Could you check a few things on this model? Use its own coordinates, in mm. Face numbers are marked on the shaded views. A direction names the side the tool comes from. Give positions to 0.01 mm unless a question says otherwise; leave off trailing zeros. Order: outer loops, then holes, each group sorted by start corner. A loop starts at its lowest first (then second) coordinate and runs counter-clockwise, first axis right, second up. Notation, with made-up numbers: (-1, -13.5) -> (42, -13.5) arc R28 cw to (42, 18.5) -> close; hole circle Ø4 at (-13.75, 62). An arc over 180 degrees is marked (long way). Answer as CSV lines item,"result". Start each with the question number.
(1) We'd pull the mould along X, two halves only. Please class the marked faces 1, 2 and 3: released by +X, released by -X, zero draft, split by the parting line, or undercut.
(2) On a 3-axis mill with a long thin cutter (end or side, diameter ignored), from which of +Z, -Z, +X, -X, +Y, -Y can I reach the whole of each face in a straight line? I mean the marked faces 4, 5 and 6. Say none if no direction works.
(3) Will these pins go through, and if not, where does the flat tip stop? pin 1 Ø14 at (y, z) = (-46.5, 30.5) entering from -X; pin 2 Ø1 at (x, y) = (91.5, -16.5) entering from +Z; pin 3 Ø3 at (x, z) = (57, 42) entering from +Y.
(4) I want a section at B-B (y = -7). Please give me the cut outline in (x, z).
(5) I want a section at C-C (z = 44.5). Please give me the cut outline in (x, y).
(6) I need wall thicknesses on L1, parallel to Z at x = 25.4, y = -32.75 (3 decimals); L2, parallel to Y at x = 40, z = 15.5; L3, parallel to X at y = -4, z = 17. Which ranges of each line are inside material? Lowest first, please.
(7) I want a section at D-D (x = 118). Please give me the cut outline in (y, z).
(8) I want a section at A-A (x = 18). Please give me the cut outline in (y, z).
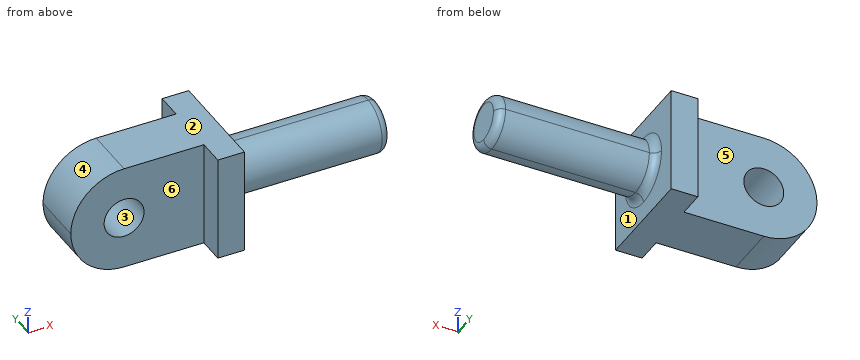
```python
from build123d import *

# Parameters (mm, degrees)
F0_W     = 76.2
F0_H     = 50.8
F1_DEPTH = 50.8
F2_W     = 63.5
F2_H     = 12.7
F3_DEPTH = 177.8
F5_DEPTH = 127
F6_R     = 25.39999
F8_DEPTH = 76.2
F9_R     = 3.81


# Not quite as in the source:
# - a fillet or chamfer is up to 0.001 mm smaller than in the source, because OpenCascade refuses the exact size


with BuildPart() as f1:
    # F0 (on Front) → F1 (new body)
    with BuildSketch(Plane.XZ):
        with Locations((38.1, 25.4)):
            Rectangle(F0_W, F0_H)
    extrude(amount=F1_DEPTH)

    # F2 (on face) → F3 (cut)
    with BuildSketch(Plane.XY.offset(50.8)):
        with Locations((31.75, -6.35)):
            Rectangle(F2_W, F2_H)
        with Locations((31.75, -44.45)):
            Rectangle(F2_W, F2_H)
    extrude(amount=-F3_DEPTH, mode=Mode.SUBTRACT)

    # F4 (on face) → F5 (cut)
    with BuildSketch(Plane.XZ.offset(38.1)):
        with BuildLine():
            ThreePointArc((15.875, 25.4), (25.4, 15.875), (34.925, 25.4))
            ThreePointArc((34.925, 25.4), (25.4, 34.925), (15.875, 25.4))
        make_face()
    extrude(amount=-F5_DEPTH, mode=Mode.SUBTRACT)

    # F6 (radius 25.4 in the source; OpenCascade refuses exactly that, so slightly less here)
    f6_edges = [f1.edges().sort_by_distance(p)[0] for p in [
        (0, -25.4, 0),
        (0, -25.4, 50.8),
    ]]
    fillet(f6_edges, radius=F6_R)

    # F7 (on face) → F8 (join)
    with BuildSketch(Plane.YZ.offset(76.2)):
        with BuildLine():
            ThreePointArc((-12.7, 25.4), (-16.4197438789, 34.3802561211), (-25.4, 38.1))
            Line((-25.4, 38.1), (-25.4, 12.7))
            ThreePointArc((-25.4, 12.7), (-16.4197438789, 16.4197438789), (-12.7, 25.4))
        make_face()
        with BuildLine():
            Line((-25.4, 12.7), (-25.4, 38.1))
            ThreePointArc((-25.4, 38.1), (-38.1, 25.4), (-25.4, 12.7))
        make_face()
    extrude(amount=F8_DEPTH)

    # F9
    f9_edges = [f1.edges().sort_by_distance(p)[0] for p in [
        (152.4, -38.1, 25.4),
        (76.2, -38.1, 25.4),
    ]]
    fillet(f9_edges, radius=F9_R)


solid = f1.part
```
Final values:
1,face 1,"released by +X"
1,face 2,"zero draft"
1,face 3,"undercut"
2,face 4,"+Z, -X, +Y, -Y"
2,face 5,"+Z, -Z, -X, +Y"
2,face 6,"+Z, -Z, -X, -Y"
3,pin 1,"x = 63.5"
3,pin 2,"z = 34.93"
3,pin 3,"y = -12.7"
4,outline,"(63.5, 0) -> (76.2, 0) -> (76.2, 50.8) -> (63.5, 50.8) -> close"
5,outline,"(8.66, -38.1) -> (63.5, -38.1) -> (63.5, -50.8) -> (76.2, -50.8) -> (76.2, 0) -> (63.5, 0) -> (63.5, -12.7) -> (8.66, -12.7) -> close"
6,L1,"0 to 15.875, 34.925 to 50.8"
6,L2,"-38.1 to -12.7"
6,L3,"63.5 to 76.2"
7,outline,"circle Ø25.4 at (-25.4, 25.4)"
8,outline,"(-38.1, 1.1) -> (-12.7, 1.1) -> (-12.7, 19.4) -> (-38.1, 19.4) -> close; (-38.1, 31.4) -> (-12.7, 31.4) -> (-12.7, 49.7) -> (-38.1, 49.7) -> close"
